Geometry check sheet. Reference: the model listing, model coordinates, mm. A direction names the side the tool comes from. Coordinates: 2 decimals unless noted, no trailing zeros. Order: outer loops, then holes, each group sorted by start corner. A loop starts at its lowest first (then second) coordinate and runs counter-clockwise, first axis right, second up. Notation, with made-up numbers: M -11.75,88.5 L 39.25,88.5 A18 cw 39.25,113.5 Z; hole C 37.25,4 d6. An arc over 180 degrees is marked long. One line per item, written item: value. Start each with the question number.
1) Thickness scan on L1, parallel to X at y = 1.8, z = -3.25; L2, parallel to Z at x = -6.75, y = 1.15; L3, parallel to Y at x = -8.75, z = 3. Record the ranges inside material, lowest first. Write a range as from..to.
2) Access from +Z, -Z, +X, -X, +Y, -Y to the whole of each face (thin tool, end or side, straight path). Record for faces 4 (the flat face through (-0.1, 2.5, 4.4)), 5 (the flat face through (-13, 2, 0)).
3) Sectioned sample at C-C, the plane x = -1.75. Enter the section's corners in (y, z).
4) Sectioned sample at A-A, the plane y = 1.7. Enter the section's corners in (x, z), then the cut area to 3 significant figures.
5) Go/stop test with a flat-tipped pin: P1, Ø1.5, axis at x = -2, z = 1.5, coming from the +Y side. Record where the tip stops, or that it passes through.
6) Sectioned sample at B-B, the plane z = 3. Enter the section's corners in (x, y), then the cut area to 3 significant figures.
7) Draft check along Z on faces 1 (the flat face through (14, 1, 0)), 2 (the flat face through (0, 1, 0)), 3 (the flat face through (0, 1, 5)). Enter one of: pulls with the +Z half, pulls with the -Z half, needs draft (parallel to the pull), parting line crosses it, or undercut.
```python
from build123d import *

# Parameters (mm, degrees)
SKETCH_1_W           = 26
SKETCH_1_H           = 8
EXTRUDE_1_DEPTH      = 1
SKETCH_2_W           = 28
SKETCH_2_H           = 10
SKETCH_2_W_2         = 26
SKETCH_2_H_2         = 8
EXTRUDE_2_DEPTH      = 1.5
EXTRUDE_2_DEPTH_BACK = 1


with BuildPart() as part:
    # 草图1 → 凸台-拉伸1 (new body)
    with BuildSketch(Plane(origin=(0, 0, 0), x_dir=(1, 0, 0), z_dir=(0, 1, 0))):
        Rectangle(SKETCH_1_W, SKETCH_1_H)
    extrude(amount=EXTRUDE_1_DEPTH)

    # 草图2 → 凸台-拉伸2 (add, two sides)
    with BuildSketch(Plane(origin=(0, 1, 0), x_dir=(1, 0, 0), z_dir=(0, 1, 0))) as extrude_2_sk:
        Rectangle(SKETCH_2_W, SKETCH_2_H)
        Rectangle(SKETCH_2_W_2, SKETCH_2_H_2, mode=Mode.SUBTRACT)
    extrude(amount=EXTRUDE_2_DEPTH)
    extrude(extrude_2_sk.sketch, amount=-EXTRUDE_2_DEPTH_BACK)


solid = part.part
```
Final values:
1. L1: x = -14..-13, 13..14
1. L2: z = -5..-4, 4..5
1. L3: y = 0..1
2. face 4: +Z, -Z, +X, -X, +Y
2. face 5: +Y
3. outline: M 0,-5 L 2.5,-5 L 2.5,-4 L 1,-4 L 1,4 L 2.5,4 L 2.5,5 L 0,5 Z
4. outline: M -14,-5 L 14,-5 L 14,5 L -14,5 Z; hole M -13,-4 L 13,-4 L 13,4 L -13,4 Z
4. area: 72.0 mm^2
5. P1: stops at y = 1
6. outline: M -14,0 L 14,0 L 14,2.5 L 13,2.5 L 13,1 L -13,1 L -13,2.5 L -14,2.5 Z
6. area: 31.0 mm^2
7. face 1: needs draft
7. face 2: undercut
7. face 3: pulls with the +Z half
